Input: part model. Units: mm. Frame: model coordinates. Round coordinates to 2 decimals unless told otherwise and drop trailing zeros. Write each loop counter-clockwise with the first axis right and the second up, starting at its lowest first coordinate (ties: lowest second). Pieces come first, ordered by that corner, then holes. Notation, with made-up numbers: (75, -22.5) - (95, -22.5) arc R21 ccw to (95, -5.5) - close; hole circle Ø1 at (54.5, -16). An arc over 180 degrees is marked (long way). One line per item, written item: value. Start each with the question number.
Autodesk Inventor part; units mm, degrees
ref_plane "Work Plane5" through (0, 0, -2) normal (0, 0, 1) x (1, 0, 0)
ref_plane "Work Plane6" through (5, 0, 0) normal (1, 0, 0) x (0, 1, 0)
ref_plane "XZ Plane" through (0, 0, 0) normal (0, 1, 0) x (-1, 0, 0)
sketch "Sketch1" plane through (0, 0, 0) normal (0, 0, 1) x (1, 0, 0)
  circle A0 centre (0, 0) radius 5
  dimension "d0" = 10
extrude "Extrusion1" add sketch "Sketch1" along normal mid plane 152.4
ref_plane "Work Plane4" through (0, 0, 0) normal (0, 0, 1) x (1, 0, 0)
ref_plane "Work Plane5" through (0, 0, -2) normal (0, 0, 1) x (1, 0, 0)
ref_plane "Work Plane6" through (5, 0, 0) normal (1, 0, 0) x (0, 1, 0)
sketch "Sketch6" plane through (5, 0, 0) normal (1, 0, 0) x (0, 1, 0)
  point P0 (0, 0)
sketch "Sketch7" plane through (5, 0, 0) normal (1, 0, 0) x (0, 1, 0)
  line L0 (0, 106.68) -> (0, -106.68)
  line L1 (-1.5, -49.2154) -> (-1.5272, -34.9251)
  line L2 (1.4728, -34.9193) -> (1.5, -49.2096)
  arc A0 (-1.5, -49.2154) -> (1.5, -49.2096) centre (0, -49.2125) ccw
  arc A1 (1.4728, -34.9193) -> (-1.5272, -34.9251) centre (-0.0272, -34.9222) ccw
  line L3 (-1.5, -49.2154) -> (1.5, -49.2096) construction
  line L4 (-1.5272, -34.9251) -> (1.4728, -34.9193) construction
  point P0 (0, 0)
  dimension "d28" = 3
extrude "Extrusion2" cut sketch "Sketch7" against normal blind 3
chamfer "Chamfer2" distance 2 angle 45 1 edges at (-5, 0, -76.2)
chamfer "Chamfer3" distance 2 angle 45 1 edges at (-5, 0, 76.2)
sketch "Sketch8" plane through (0, 0, 76.2) normal (0, 0, 1) x (1, 0, 0)
  circle A0 centre (0, 0) radius 1
  dimension "d48" = 2
extrude "Extrusion3" add sketch "Sketch8" along normal blind 6
fillet "Fillet1" radius 0.2 1 edges at (-1, 0, 82.2)
sketch "Sketch9" plane through (0, 0, 0) normal (1, 0, 0) x (0, 1, 0)
  line L0 (-5, -74.2) -> (5, -74.2)
  line L1 (-1.5, -49.2154) -> (-1.5272, -34.9251)
  line L2 (1.4728, -34.9193) -> (1.5, -49.2096)
  line L3 (5, 74.2) -> (-5, 74.2)
  line L4 (-5, -74.2) -> (-5, 74.2)
  circle A0 centre (-5, -69.85) radius 1
  circle A1 centre (-5, -23.8125) radius 0.75
  line L5 (0, -103.88) -> (0, 103.88)
  point P0 (0, 0)
  point P1 (0, -50.7125)
  point P2 (0, -33.4224)
  dimension "d53" = 2
  dimension "d54" = 1.5
revolve "Revolution4" cut sketch "Sketch9" angle 360 about axis through (0, 0, -10) along (0, 0, 1) contours A0 L4 | L4 A0 | A1 L4 | L4 A1
properties part number "Motor shaft" material "Steel, High Strength Low Alloy"
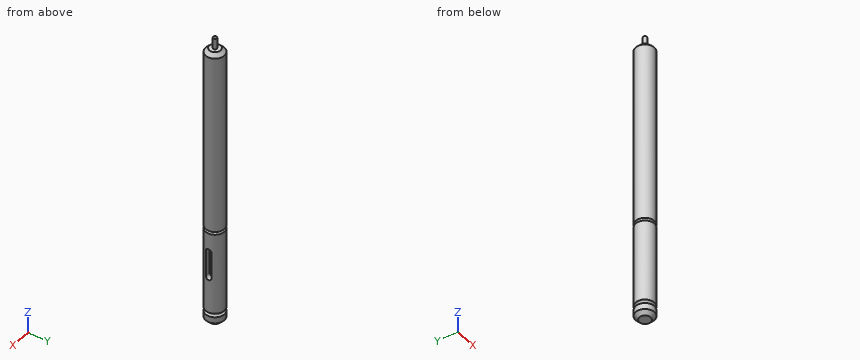
Q1. Cut plane B-B, the plane z = -41.5. Output: boundary loops of the cut face in (x, y).
Q2. Material intervals for probe 1 along Z at (x, y) = (2.25, 0); probe 2 along Z at (x, y) = (-3, 3.5); probe 3 along Z at (x, y) = (-3, -3.25), sorted ascending. Write a range as from..to.
Q3. Contact query for flat-ended pins moving along their axis: pin 1 Ø4 at (x, z) = (2, 9.5) entering from +Y; pin 2 Ø1.5 at (y, z) = (0, -43) entering from +X. Output: stop coordinate, or through.
Q4. Cut plane A-A, the plane z = 26.5. Output: boundary loops of the cut face in (x, y).
A:
1. outline: (2, -1.51) - (2, 1.49) - (4.77, 1.49) arc R5 ccw (long way) to (4.77, -1.51) - close
2. probe 1: z = -76.2..-50.71, -33.42..76.2
2. probe 2: z = -74.59..-70.77, -68.93..-24.45, -23.17..74.59
2. probe 3: z = -74.78..-70.67, -69.03..-24.29, -23.33..74.78
3. pin 1: stops at y = 5
3. pin 2: stops at x = 2
4. outline: circle Ø10 at (0, 0)
